Job drawing, mm, ordinate dimensions from the low corner. One solid piece. Give positions to 0.01 mm unless a question says otherwise; leave off trailing zeros. Order: outer loops, then holes, each group sorted by start corner. A loop starts at its lowest first (then second) coordinate and runs counter-clockwise, first axis right, second up. Notation, with made-up numbers: M 20.5,48.5 L 29.5,48.5 A21 ccw 29.5,78.5 Z; hole C 7,-29 d8. An arc over 180 degrees is marked long. Use CSV: the item, a comma, the result in double quotes. Start each with the question number.
Item 1: Wall check: line 1 along Z through (x, y) = (30, 44.45); line 2 along Y through (x, z) = (27, 44). Give the ranges that are in metal, low to high.
Item 2: Band-saw the part on A-A on y = 44.45. Write the cut outline in (x, z).
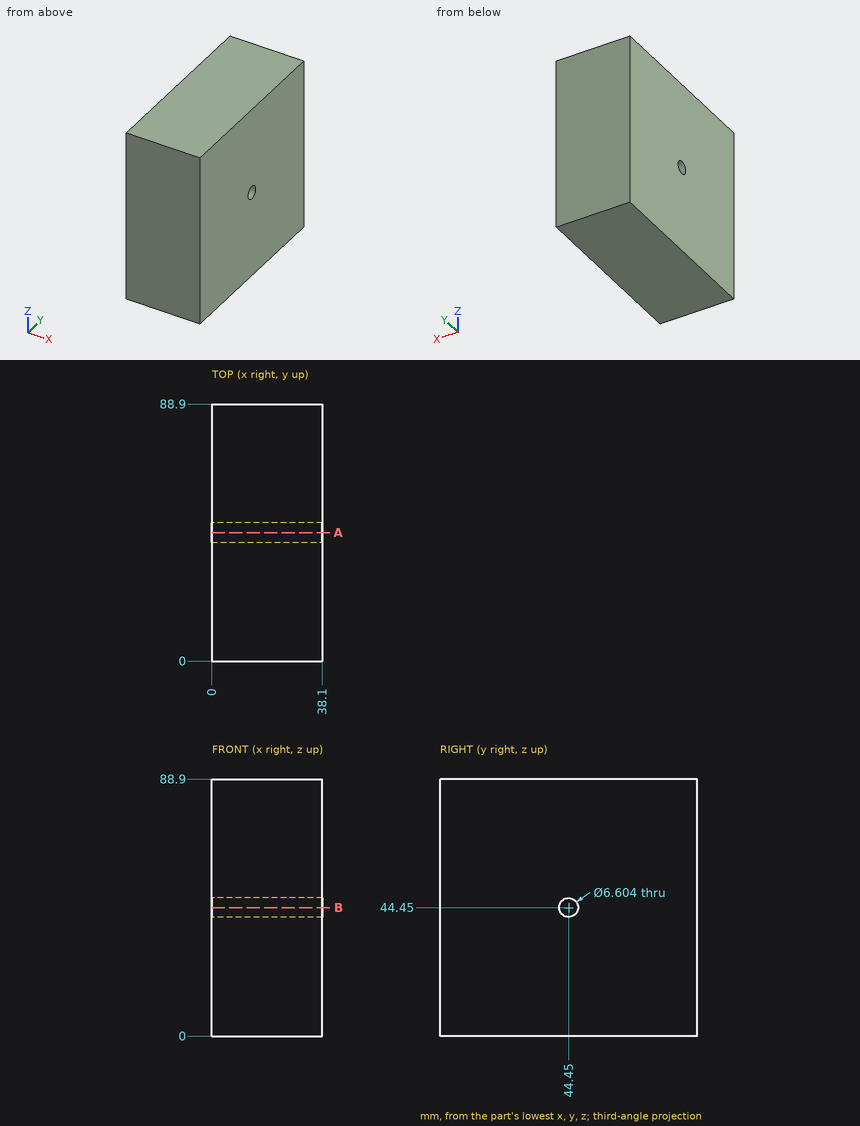
Model answer:
1,line 1,"z = 0 to 41.15, 47.75 to 88.9"
1,line 2,"y = 0 to 41.18, 47.72 to 88.9"
2,outline,"M 0,0 L 38.1,0 L 38.1,41.15 L 0,41.15 Z; M 0,47.75 L 38.1,47.75 L 38.1,88.9 L 0,88.9 Z"
